```python
from build123d import *

# Parameters (mm, degrees)
F0_W     = 77.8
F0_H     = 171.8
F0_R     = 16
F1_DEPTH = 57


with BuildPart() as f1:
    # F0 (on Right) → F1 (new body)
    with BuildSketch(Plane.YZ):
        Rectangle(F0_W, F0_H)
        Circle(F0_R, mode=Mode.SUBTRACT)
    extrude(amount=F1_DEPTH)


solid = f1.part
```
Can you work these out from the model? Positions are in its coordinate system, mm. Give positions to 0.01 mm unless a question says otherwise; leave off trailing zeros. Loops run counter-clockwise (first coordinate to the right, second up) from the corner with the lowest first, then second, coordinate; pieces in that order, holes last. Notation, with made-up numbers: M 30.25,-29.75 L 56.25,-29.75 A26 ccw 56.25,-13.75 Z; hole C 31,63.5 d7. An arc over 180 degrees is marked long. Use CSV: the item, a comma, the result in double quotes. Start each with the question number.
1. Imagine slicing it at C-C, the plane x = 18.5. Write out the boundary of the cut face in (y, z), plus the area to 3 significant figures.
2. Imagine slicing it at A-A, the plane y = 0. Write out the boundary of the cut face in (x, z).
3. If we mould it in two halves opening along Y, with no side actions, what happens to faces 1 (the face through (28.1, -3.47, -15.62)), 2 (the face through (28, -38.9, -1)), 3 (the face through (57, 17, 1)), 4 (the face through (28, 38.9, -1))? For each: released by +Y, released by -Y, zero draft, split by the parting line, or undercut.
4. Imagine slicing it at B-B, the plane z = 0. Write out the boundary of the cut face in (x, y), plus the area to 3 significant figures.
5. If I drill on L1, parallel to Z at x = 36.5, y = 0; L2, parallel to Z at x = 10.5, y = 13, over which ranges is the centre line in solid material (lowest first)?
Response values:
1,outline,"M -38.9,-85.9 L 38.9,-85.9 L 38.9,85.9 L -38.9,85.9 Z; hole C 0,0 d32"
1,area,"12,600 mm^2"
2,outline,"M 0,-85.9 L 57,-85.9 L 57,-16 L 0,-16 Z; M 0,16 L 57,16 L 57,85.9 L 0,85.9 Z"
3,face 1,"undercut"
3,face 2,"released by -Y"
3,face 3,"zero draft"
3,face 4,"released by +Y"
4,outline,"M 0,-38.9 L 57,-38.9 L 57,-16 L 0,-16 Z; M 0,16 L 57,16 L 57,38.9 L 0,38.9 Z"
4,area,"2,610 mm^2"
5,L1,"-85.9 to -16, 16 to 85.9"
5,L2,"-85.9 to -9.33, 9.33 to 85.9"
